Autodesk Inventor part; units mm, degrees
ref_plane "YZ Plane" through (0, 0, 0) normal (1, 0, 0) x (0, 1, 0)
ref_plane "XZ Plane" through (0, 0, 0) normal (0, 1, 0) x (-1, 0, 0)
ref_plane "XY Plane" through (0, 0, 0) normal (0, 0, 1) x (1, 0, 0)
sketch "Sketch1" plane through (0, 0, 0) normal (0, 0, 1) x (1, 0, 0)
  circle A0 centre (0, 0) radius 2.1
  circle A1 centre (20, 0) radius 2.1
  circle A2 centre (40, 0) radius 2.1
  line L0 (0, 0) -> (40, 0) construction
  line L1 (0, 0) -> (40, 0) construction
  line L2 (0, -4) -> (40, -4)
  line L3 (40, 4) -> (0, 4)
  arc A3 (0, 4) -> (0, -4) centre (0, 0) ccw
  arc A4 (40, -4) -> (40, 4) centre (40, 0) ccw
  dimension "d0" = 4.2
  dimension "d1" = 4.2
  dimension "d2" = 4.2
  dimension "d3" = 20
  dimension "d4" = 20
  dimension "d5" = 0
  dimension "d6" = 8
extrude "Extrusion1" add sketch "Sketch1" against normal blind 30
properties part number "battery_top_secure"
Input: part model. Units: mm. Frame: model coordinates. Round coordinates to 2 decimals unless told otherwise and drop trailing zeros. Loops run counter-clockwise (first coordinate to the right, second up) from the corner with the lowest first, then second, coordinate; pieces in that order, holes last. Notation, with made-up numbers: (71, -26) -> (81, -26) arc R22 cw to (81, -18) -> close; hole circle Ø7 at (86, 45). An arc over 180 degrees is marked (long way). Write each question's results on one line, items separated by ' | '.
1. Ray query, line 1 (Y direction, x = 40, z = -12.5); line 2 (X direction, y = 1.5, z = -11.5); line 3 (X direction, y = -1, z = -7.5). Return the intervals inside material, ascending. Write a range as from..to.
Geometry results:
line 1: -4..-2.1, 2.1..4 | line 2: -3.71..-1.47, 1.47..18.53, 21.47..38.53, 41.47..43.71 | line 3: -3.87..-1.85, 1.85..18.15, 21.85..38.15, 41.85..43.87
2. Section A-A (y = 0). Return loops of the section in (x, z), and give its area (3 significant figures).
Geometry results:
outline: (-4, -30) -> (-2.1, -30) -> (-2.1, 0) -> (-4, 0) -> close; (2.1, -30) -> (17.9, -30) -> (17.9, 0) -> (2.1, 0) -> close; (22.1, -30) -> (37.9, -30) -> (37.9, 0) -> (22.1, 0) -> close; (42.1, -30) -> (44, -30) -> (44, 0) -> (42.1, 0) -> close | area: 1,060 mm2
3. Section B-B (z = -22.5). Return loops of the section in (x, y).
Geometry results:
outline: (0, -4) -> (40, -4) arc R4 ccw to (40, 4) -> (0, 4) arc R4 ccw to start; hole circle Ø4.2 at (0, 0); hole circle Ø4.2 at (20, 0); hole circle Ø4.2 at (40, 0)
4. Section C-C (y = 3). Return loops of the section in (x, z), and give its area (3 significant figures).
Geometry results:
outline: (-2.65, -30) -> (42.65, -30) -> (42.65, 0) -> (-2.65, 0) -> close | area: 1,360 mm2
5. First-contact query: P1, Ø1, axis at y = -1, z = -4, coming from the -X side; P2, Ø2, axis at y = -3, z = -7.5, coming from the +X side; P3, Ø1.5, axis at x = 6.5, y = 1.5, coming from the +Z side. Flat tips, straight axial feed; report the tip coordinate or a pass-through.
Geometry results:
P1: x = -3.97 | P2: x = 43.46 | P3: z = 0
6. Mould query, pull axis X, two halves, no side actions, for faces 1 (the face through (20, 4, -15)), 2 (the face through (44, 0, -15)), 3 (the face through (22.003, 0.631, -14.79)). Classes: +X half, -X half, draft (parallel to the pull), parting line (faces both ways), or undercut.
Geometry results:
face 1: draft | face 2: +X half | face 3: undercut
